Verification items for the finished model (mm, model axes). A direction names the side the tool comes from. Give positions to 0.01 mm unless a question says otherwise; leave off trailing zeros. Order: outer loops, then holes, each group sorted by start corner. A loop starts at its lowest first (then second) coordinate and runs counter-clockwise, first axis right, second up. Notation, with made-up numbers: M 6.5,57 L 58.5,57 A21 cw 58.5,87 Z; hole C 74,8 d11. An arc over 180 degrees is marked long. Answer as a JSON object with one key per item and string values.
```python
from build123d import *

# Parameters (mm, degrees)
PAD_DEPTH           = 74
SKETCH001_W         = 13
SKETCH001_H         = 6
POCKET_DEPTH        = 8
LINEARPATTERN_COUNT = 2
LINEARPATTERN_PITCH = 19
SKETCH002_R         = 2.836223
SKETCH002_W         = 6.476894
SKETCH002_H         = 2.419083
SKETCH002_W_2       = 7.491354
SKETCH002_H_2       = 2.106944
POCKET001_DEPTH     = 5


with BuildPart() as part:
    # Sketch → Pad (new body, symmetric)
    with BuildSketch(Plane.YZ):
        with BuildLine():
            ThreePointArc((-31.68, 7.7), (-36.68, 0), (-31.68, -7.7))
            Line((-31.68, -7.7), (31.68, -7.7))
            ThreePointArc((31.68, -7.7), (36.68, 0), (31.68, 7.7))
            Line((-31.68, 7.7), (31.68, 7.7))
        make_face()
    extrude(amount=PAD_DEPTH, both=True)

    # Sketch001 (on DatumPlane) → Pocket (cut)
    with BuildSketch(Plane.YZ.offset(74)):
        with Locations((-23.331998, 0.508297)):
            Rectangle(SKETCH001_W, SKETCH001_H)
    pocket = extrude(amount=-POCKET_DEPTH, mode=Mode.SUBTRACT)

    # LinearPattern: Pocket ×2
    with Locations(*[(0, i * LINEARPATTERN_PITCH, 0) for i in range(1, LINEARPATTERN_COUNT)]):
        add(pocket, mode=Mode.SUBTRACT)

    # Sketch002 (on DatumPlane) → Pocket001 (cut)
    with BuildSketch(Plane.YZ.offset(74)):
        with Locations((29.637125, 0)):
            Circle(SKETCH002_R)
        with Locations((8.216534, 2.288247)):
            Rectangle(SKETCH002_W, SKETCH002_H)
        with Locations((17.931886, 2.210213)):
            Rectangle(SKETCH002_W_2, SKETCH002_H_2)
    extrude(amount=-POCKET001_DEPTH, mode=Mode.SUBTRACT)


solid = part.part
```
Q1. Gauge pin test, flat ends, axial feed: pin 1 Ø1.5 at (x, z) = (40, -4.5) entering from -Y; pin 2 Ø1.9 at (x, z) = (71.5, 2.5) entering from +Y; pin 3 Ø2.5 at (x, z) = (70.5, 2) entering from -Y. Record the tip position at first contact, or that the pin passes through.
Resolved:
{"pin 1": "stops at y = -35.8", "pin 2": "stops at y = 36.54", "pin 3": "stops at y = -36.65"}
Q2. Section check B-B on x = -62.5. Record the cut outline in (y, z), then the cut area to 3 significant figures.
Resolved:
{"outline": "M -31.68,-7.7 L 31.68,-7.7 A8.43 ccw 31.68,7.7 L -31.68,7.7 A8.43 ccw Z", "area": "1,090 mm²"}
Q3. Section check A-A on y = -26. Record the cut outline in (x, z).
Resolved:
{"outline": "M -74,-7.7 L 74,-7.7 L 74,-2.49 L 66,-2.49 L 66,3.51 L 74,3.51 L 74,7.7 L -74,7.7 Z"}
Q4. Tool access check on faces 1 (the face through (1.04, -36.68, 0.14)), 2 (the face through (70, -23, -2.492)). Record the directions out of +Z, -Z, +X, -X, +Y, -Y that give a thin tool (end or side, any length) a straight path to the whole face; none if there is none.
Resolved:
{"face 1": "+X, -X, -Y", "face 2": "+X"}
Q5. Release check for a two-part mould opening along Y. For faces 3 (the face through (69, 30, 0)), 4 (the face through (1, 0, 7.7)), 5 (the face through (71.535, 26.804, 0.125)), 6 (the face through (1.04, 36.68, -0.14)) record: +Y half, -Y half, draft (parallel to the pull), parting line (faces both ways), or undercut.
Resolved:
{"face 3": "undercut", "face 4": "draft", "face 5": "undercut", "face 6": "+Y half"}
Q6. Section check C-C on z = -5.25. Record the cut outline in (x, y).
Resolved:
{"outline": "M -74,-34.85 L 74,-34.85 L 74,34.85 L -74,34.85 Z"}
Q7. Material ranges on L1, parallel to X at y = -20, z = -1.75; L2, parallel to Y at x = 1.5, z = 0.25; L3, parallel to Y at x = 46, z = 6.5, recorded low to high.
Resolved:
{"L1": "x = -74 to 66", "L2": "y = -36.68 to 36.68", "L3": "y = -33.62 to 33.62"}
